Design review of the part built by this model. Coordinates are the model's own, in mm. Coordinates: 2 decimals unless noted, no trailing zeros. Loops run counter-clockwise (first coordinate to the right, second up) from the corner with the lowest first, then second, coordinate; pieces in that order, holes last. Notation, with made-up numbers: (47.25, 40) - (51.25, 40) arc R16 cw to (51.25, 56) - close; hole circle Ø10 at (60, 74). An arc over 180 degrees is marked (long way). Use one line per item in the form item = value. Start each with the question number.
(1) For L1, parallel to Z at x = 16.25, y = 399; L2, parallel to Y at x = 3.5, z = -198; L3, parallel to Y at x = 15.5, z = -241.5, list the stretches that pass through material, from the lowest coordinate up.
(2) The part is to be moulded in two halves that separate along Z. For faces 1 (the face through (11.65, 286.3, -45.5)), 2 (the face through (0, 289, -197)), 3 (the face through (6, 281, -376.55)), say which applies: pulls with the +Z half, pulls with the -Z half, needs draft (parallel to the pull), parting line crosses it, or undercut.
(3) Clearance check with flat-ended pins moving along their axes: pin 1 Ø1 at (x, z) = (13, -127.5) entering from -Y; pin 2 Ø7 at (x, y) = (16, 328) entering from -Z; pin 3 Ø3 at (x, z) = (15.5, -216) entering from +Y. State where each tip first meets the part, or that it passes through.
(4) Add section B-B (z = -313.5). State the section outline as (x, y) points (3 decimals).
(5) Add section A-A (y = 515). State the section outline as (x, z) points (3 decimals), plus the area to 3 significant figures.
```python
from build123d import *

# Parameters (mm, degrees)
SKETCH1_W           = 376.55000001
SKETCH1_H           = 570
BOSS_EXTRUDE1_DEPTH = 18
SKETCH5_W           = 18
SKETCH5_H           = 557.3
CUT_EXTRUDE3_DEPTH  = 6.35
SKETCH7_W           = 376.55000001
SKETCH7_H           = 18
CUT_EXTRUDE4_DEPTH  = 6.35
FILLET1_R           = 9.525
SKETCH9_W           = 19.05
SKETCH9_H           = 534
CUT_EXTRUDE6_DEPTH  = 6.35
SKETCH10_W          = 12.7
SKETCH10_H          = 570
CUT_EXTRUDE7_DEPTH  = 19
FILLET2_R           = 9.525
SKETCH11_R          = 1.7859375
CUT_EXTRUDE8_DEPTH  = 12.65


with BuildPart() as part:
    # Sketch1 → Boss-Extrude1 (new body)
    with BuildSketch(Plane(origin=(0, 0, 0), x_dir=(0, 0, -1), z_dir=(1, 0, 0))):
        with Locations((188.275000005, 285)):
            Rectangle(SKETCH1_W, SKETCH1_H)
    extrude(amount=BOSS_EXTRUDE1_DEPTH)

    # Sketch5 → Cut-Extrude3 (cut)
    with BuildSketch(Plane(origin=(18, 0, 0), x_dir=(0, 0, -1), z_dir=(1, 0, 0))):
        with Locations((47.1, 285)):
            Rectangle(SKETCH5_W, SKETCH5_H)
    extrude(amount=-CUT_EXTRUDE3_DEPTH, mode=Mode.SUBTRACT)

    # Sketch7 → Cut-Extrude4 (cut)
    with BuildSketch(Plane(origin=(18, 0, 0), x_dir=(0, 0, -1), z_dir=(1, 0, 0))):
        with Locations((188.275000005, 9)):
            Rectangle(SKETCH7_W, SKETCH7_H)
        with Locations((188.275000005, 561)):
            Rectangle(SKETCH7_W, SKETCH7_H)
    extrude(amount=-CUT_EXTRUDE4_DEPTH, mode=Mode.SUBTRACT)

    # Fillet1
    fillet1_edges = [part.edges().sort_by_distance(p)[0] for p in [
        (5.825, 0, 0),
        (0, 570, -188.275000005),
        (0, 0, -188.275000005),
        (5.825, 570, 0),
        (0, 285, 0),
    ]]
    fillet(fillet1_edges, radius=FILLET1_R)

    # Sketch9 → Cut-Extrude6 (cut)
    with BuildSketch(Plane(origin=(18, 0, 0), x_dir=(0, 0, -1), z_dir=(1, 0, 0))):
        with Locations((367.02500001, 285)):
            Rectangle(SKETCH9_W, SKETCH9_H)
    extrude(amount=-CUT_EXTRUDE6_DEPTH, mode=Mode.SUBTRACT)

    # Sketch10 → Cut-Extrude7 (cut, through all)
    with BuildSketch(Plane(origin=(18, 0, 0), x_dir=(0, 0, -1), z_dir=(1, 0, 0))):
        with Locations((6.35, 285)):
            Rectangle(SKETCH10_W, SKETCH10_H)
    extrude(amount=-CUT_EXTRUDE7_DEPTH, mode=Mode.SUBTRACT)

    # Fillet2
    fillet2_edges = [part.edges().sort_by_distance(p)[0] for p in [
        (2.789807909, 2.789807909, -12.7),
        (0, 285, -12.7),
        (10.5875, 570, -12.7),
        (2.789807909, 567.210192091, -12.7),
        (10.5875, 0, -12.7),
    ]]
    fillet(fillet2_edges, radius=FILLET2_R)

    # Sketch11 → Cut-Extrude8 (cut, through all)
    with BuildSketch(Plane(origin=(11.65, 0, 0), x_dir=(0, 0, -1), z_dir=(1, 0, 0))):
        with Locations((47.625, 285)):
            Circle(SKETCH11_R)
        with Locations((47.625, 560.475)):
            Circle(SKETCH11_R)
        with Locations((199.387500005, 560.475)):
            Circle(SKETCH11_R)
        with Locations((367.02500001, 560.475)):
            Circle(SKETCH11_R)
        with Locations((367.02500001, 285)):
            Circle(SKETCH11_R)
        with Locations((367.02500001, 9.525)):
            Circle(SKETCH11_R)
        with Locations((199.387500005, 9.525)):
            Circle(SKETCH11_R)
        with Locations((47.625, 9.525)):
            Circle(SKETCH11_R)
        with Locations((47.625, 34.925)):
            Circle(SKETCH11_R)
        with Locations((367.02500001, 34.925)):
            Circle(SKETCH11_R)
        with Locations((47.625, 535.075)):
            Circle(SKETCH11_R)
        with Locations((367.02500001, 535.075)):
            Circle(SKETCH11_R)
    extrude(amount=-CUT_EXTRUDE8_DEPTH, mode=Mode.SUBTRACT)


solid = part.part
```
Computed values:
q1.L1 = -357.5 to -56.1, -38.1 to -12.7
q1.L2 = 2.15 to 8.4, 10.65 to 559.35, 561.6 to 567.85
q1.L3 = 18 to 552
q2.face_1 = undercut
q2.face_2 = needs draft
q2.face_3 = pulls with the -Z half
q3.pin_1 = 18
q3.pin_2 = -357.5
q3.pin_3 = 552
q4.outline = (0, 9.525) arc R9.525 ccw to (9.525, 0) - (11.65, 0) - (11.65, 18) - (18, 18) - (18, 552) - (11.65, 552) - (11.65, 570) - (9.525, 570) arc R9.525 ccw to (0, 560.475) - close
q5.outline = (0, -376.55) - (11.65, -376.55) - (11.65, -357.5) - (18, -357.5) - (18, -56.1) - (11.65, -56.1) - (11.65, -38.1) - (18, -38.1) - (18, -12.7) - (9.525, -12.7) arc R9.525 ccw to (0, -22.225) - close
q5.area = 6,290 mm^2
